Geometry check sheet. Reference: the model listing, model coordinates, mm. A direction names the side the tool comes from. Round coordinates to 2 decimals unless told otherwise and drop trailing zeros. Write each loop counter-clockwise with the first axis right and the second up, starting at its lowest first coordinate (ties: lowest second). Pieces come first, ordered by that corner, then holes. Notation, with made-up numbers: (72, 71) -> (105, 71) arc R24 cw to (105, 99) -> close; hole circle Ø5 at (27.25, -37.75). An arc over 180 degrees is marked (long way). One line per question, with ' | ' between items.
```python
from build123d import *

# Parameters (mm, degrees)
SKETCH1_W           = 200
SKETCH1_H           = 70
BOSS_EXTRUDE1_DEPTH = 100
SKETCH2_W           = 20
SKETCH2_H           = 50
BOSS_EXTRUDE3_DEPTH = 50
SKETCH3_W           = 25
SKETCH3_H           = 30
CUT_EXTRUDE1_DEPTH  = 25
SKETCH4_R           = 2.5
CUT_EXTRUDE2_DEPTH  = 15
SKETCH5_R           = 3.75
CUT_EXTRUDE3_DEPTH  = 4
SKETCH6_R           = 2
CUT_EXTRUDE4_DEPTH  = 15
SKETCH7_W           = 180
SKETCH7_H           = 62
CUT_EXTRUDE5_DEPTH  = 60
SKETCH8_R           = 2
CUT_EXTRUDE6_DEPTH  = 15
SKETCH9_R           = 2.5
CUT_EXTRUDE7_DEPTH  = 168.332005307
SKETCH10_R          = 3.75
CUT_EXTRUDE8_DEPTH  = 4


with BuildPart() as part:
    # Sketch1 → Boss-Extrude1 (new body)
    with BuildSketch(Plane(origin=(0, 0, 0), x_dir=(1, 0, 0), z_dir=(0, 1, 0))):
        Rectangle(SKETCH1_W, SKETCH1_H)
    extrude(amount=BOSS_EXTRUDE1_DEPTH)

    # Sketch2 → Boss-Extrude3 (add)
    with BuildSketch(Plane(origin=(0, 100, 0), x_dir=(1, 0, 0), z_dir=(0, 1, 0))):
        with Locations((-110, 2.5)):
            Rectangle(SKETCH2_W, SKETCH2_H)
        with Locations((110, 2.5)):
            Rectangle(SKETCH2_W, SKETCH2_H)
    extrude(amount=-BOSS_EXTRUDE3_DEPTH)

    # Sketch3 → Cut-Extrude1 (cut)
    with BuildSketch(Plane.XZ):
        with Locations((77.5, -15)):
            Rectangle(SKETCH3_W, SKETCH3_H)
        with Locations((-77.5, -15)):
            Rectangle(SKETCH3_W, SKETCH3_H)
    extrude(amount=-CUT_EXTRUDE1_DEPTH, mode=Mode.SUBTRACT)

    # Sketch4 → Cut-Extrude2 (cut)
    with BuildSketch(Plane(origin=(0, 0, -35), x_dir=(-1, 0, 0), z_dir=(0, 0, -1))):
        with Locations((-77.5, 12.5)):
            Circle(SKETCH4_R)
        with Locations((77.5, 12.5)):
            Circle(SKETCH4_R)
    extrude(amount=-CUT_EXTRUDE2_DEPTH, mode=Mode.SUBTRACT)

    # Sketch5 → Cut-Extrude3 (cut)
    with BuildSketch(Plane(origin=(0, 0, -35), x_dir=(-1, 0, 0), z_dir=(0, 0, -1))):
        with Locations((-77.5, 12.5)):
            Circle(SKETCH5_R)
        with Locations(Location((77.5, 12.5, 0), (0, 0, 180))):
            Circle(SKETCH5_R)
    extrude(amount=-CUT_EXTRUDE3_DEPTH, mode=Mode.SUBTRACT)

    # Sketch6 → Cut-Extrude4 (cut)
    with BuildSketch(Plane(origin=(0, 0, -27.5), x_dir=(-1, 0, 0), z_dir=(0, 0, -1))):
        with Locations((-110, 87.5)):
            Circle(SKETCH6_R)
        with Locations(Location((-110, 62.5, 0), (0, 0, 180))):
            Circle(SKETCH6_R)
        with Locations((110, 62.5)):
            Circle(SKETCH6_R)
        with Locations(Location((110, 87.5, 0), (0, 0, 180))):
            Circle(SKETCH6_R)
    extrude(amount=-CUT_EXTRUDE4_DEPTH, mode=Mode.SUBTRACT)

    # Sketch7 → Cut-Extrude5 (cut)
    with BuildSketch(Plane(origin=(0, 0, -35), x_dir=(-1, 0, 0), z_dir=(0, 0, -1))):
        with Locations((0, 59)):
            Rectangle(SKETCH7_W, SKETCH7_H)
    extrude(amount=-CUT_EXTRUDE5_DEPTH, mode=Mode.SUBTRACT)

    # Sketch8 → Cut-Extrude6 (cut)
    with BuildSketch(Plane(origin=(0, 0, -35), x_dir=(-1, 0, 0), z_dir=(0, 0, -1))):
        with Locations((-45, 15)):
            Circle(SKETCH8_R)
        with Locations(Location((45, 15, 0), (0, 0, 180))):
            Circle(SKETCH8_R)
        with Locations((-93, 93)):
            Circle(SKETCH8_R)
        with Locations(Location((93, 93, 0), (0, 0, 180))):
            Circle(SKETCH8_R)
    extrude(amount=-CUT_EXTRUDE6_DEPTH, mode=Mode.SUBTRACT)

    # Sketch9 → Cut-Extrude7 (cut, through all)
    with BuildSketch(Plane(origin=(0, 0, 25), x_dir=(-1, 0, 0), z_dir=(0, 0, -1))):
        with Locations((-55, 80)):
            Circle(SKETCH9_R)
        with Locations(Location((55, 80, 0), (0, 0, 180))):
            Circle(SKETCH9_R)
        with Locations((55, 38)):
            Circle(SKETCH9_R)
        with Locations(Location((-55, 38, 0), (0, 0, 180))):
            Circle(SKETCH9_R)
    extrude(amount=-CUT_EXTRUDE7_DEPTH, mode=Mode.SUBTRACT)

    # Sketch10 → Cut-Extrude8 (cut)
    with BuildSketch(Plane(origin=(0, 0, 25), x_dir=(-1, 0, 0), z_dir=(0, 0, -1))):
        with Locations((-55, 80)):
            Circle(SKETCH10_R)
        with Locations(Location((-55, 38, 0), (0, 0, 180))):
            Circle(SKETCH10_R)
        with Locations((55, 38)):
            Circle(SKETCH10_R)
        with Locations(Location((55, 80, 0), (0, 0, 180))):
            Circle(SKETCH10_R)
    extrude(amount=-CUT_EXTRUDE8_DEPTH, mode=Mode.SUBTRACT)


solid = part.part
```
(1) Sectioned sample at D-D on z = -17. Record the cut outline in (x, y), then the cut area to 3 significant figures.
Resolved:
outline: (-120, 50) -> (-100, 50) -> (-100, 0) -> (-90, 0) -> (-90, 25) -> (-65, 25) -> (-65, 0) -> (65, 0) -> (65, 25) -> (90, 25) -> (90, 0) -> (100, 0) -> (100, 50) -> (120, 50) -> (120, 100) -> (-120, 100) -> close; hole circle Ø4 at (-110, 62.5); hole circle Ø4 at (-110, 87.5); hole (-90, 28) -> (90, 28) -> (90, 90) -> (-90, 90) -> close; hole circle Ø4 at (110, 62.5); hole circle Ø4 at (110, 87.5) | area: 9,540 mm2
(2) Sectioned sample at B-B on z = 7. Record the cut outline in (x, y).
Resolved:
outline: (-120, 50) -> (-100, 50) -> (-100, 0) -> (100, 0) -> (100, 50) -> (120, 50) -> (120, 100) -> (-120, 100) -> close; hole (-90, 28) -> (90, 28) -> (90, 90) -> (-90, 90) -> close
(3) Sectioned sample at A-A on y = 80. Count the separate pieces of the cut face and the enclosed holes in it, then the cut area to 3 significant figures.
Resolved:
separate pieces: 3 | enclosed holes: 0 | area: 5,080 mm2
(4) Draft check along Z on faces 4 (the flat face through (58, 80, 29)), 5 (the flat face through (77, 25, -15)), 6 (the cylindrical face through (-58.464, 36.564, 26.972)). Enter one of: +Z half, -Z half, draft (parallel to the pull), parting line (faces both ways), or undercut.
Resolved:
face 4: -Z half | face 5: undercut | face 6: draft
(5) Go/stop test with flat-tipped pins: pin 1 (8 mm diameter, centred on x = -77.5, y = 14, fed in from -Z); pin 2 (2.5 mm diameter, centred on x = -45, y = 15, fed in from -Z); pin 3 (7.5 mm diameter, centred on y = 9, z = -21.5, fed in from -X); pin 4 (10 mm diameter, centred on x = -113.5, y = 86.5, fed in from +Z). Record where each tip stops, or that it passes through.
Resolved:
pin 1: stops at z = -35 | pin 2: stops at z = -20 | pin 3: stops at x = -100 | pin 4: stops at z = 22.5
(6) Access from +Z, -Z, +X, -X, +Y, -Y to the whole of each face (thin tool, end or side, straight path). Record for faces 1 (the flat face through (110, 50, -3)), 2 (the flat face through (1, 59, 25)), 3 (the flat face through (77, 12, 0)).
Resolved:
face 1: +Z, -Z, +X, -Y | face 2: -Z | face 3: -Y
(7) Sectioned sample at C-C on x = -55. Record the cut outline in (y, z), then the cut area to 3 significant figures.
Resolved:
outline: (0, -35) -> (28, -35) -> (28, 25) -> (34.25, 25) -> (34.25, 29) -> (35.5, 29) -> (35.5, 35) -> (0, 35) -> close; (40.5, 29) -> (41.75, 29) -> (41.75, 25) -> (76.25, 25) -> (76.25, 29) -> (77.5, 29) -> (77.5, 35) -> (40.5, 35) -> close; (82.5, 29) -> (83.75, 29) -> (83.75, 25) -> (90, 25) -> (90, -35) -> (100, -35) -> (100, 35) -> (82.5, 35) -> close | area: 3,160 mm2
(8) Material ranges on line 1 (Y direction, x = -55, z = 27.25); line 2 (Z direction, x = 67, y = 10); line 3 (Y direction, x = -58.5, z = 14), recorded low to high.
Resolved:
line 1: y = 0 to 34.25, 41.75 to 76.25, 83.75 to 100 | line 2: z = -35 to -30, 0 to 35 | line 3: y = 0 to 28, 90 to 100
